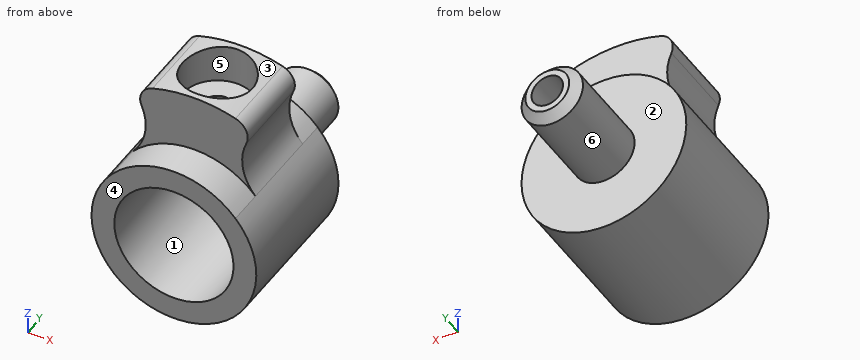
```python
from build123d import *

# Parameters (mm, degrees)
CUT_EXTRUDE_1_DEPTH   = 9.2
FILLET_1_R            = 1
SKETCH_5_OUTSIDE_W    = 15.602
SKETCH_5_OUTSIDE_H    = 18.902
SKETCH_5_OUTSIDE_R    = 4.7
CUT_EXTRUDE_4_DEPTH   = 1.5
CUT_EXTRUDE_START     = -8.2
SKETCH_5_2_OUTSIDE_W  = 15.602
SKETCH_5_2_OUTSIDE_H  = 18.902
SKETCH_5_2_OUTSIDE_R  = 4.7
CUT_EXTRUDE_5_DEPTH   = 2
CHAMFER_1_SIZE        = 0.5
M2_TAPPED_HOLE1_D     = 1.6
M2_TAPPED_HOLE1_DEPTH = 5.2
M2_TAPPED_HOLE1_TIP   = 0.480688495
SKETCH4_R             = 2
CUT_EXTRUDE1_DEPTH    = 2.2


with BuildPart() as part:
    # Эскиз1 → Повернуть1 (revolve)
    with BuildSketch(Plane(origin=(0, 0, 0), x_dir=(0, 0, -1), z_dir=(1, 0, 0))):
        Polygon((-3.4, 0), (-3.4, 6.5), (-0.9, 6.5), (-0.9, 13.85), (-1.75, 13.85), (-1.75, 8.2), (-8, 8.2), (-8, 0), align=None)
    revolve(axis=Axis((0, 0, 0), (0, 1, 0)))

    # Эскиз2 → Вырез-Вытянуть1 (cut, through all)
    with BuildSketch(Plane(origin=(0, 8.2, 0), x_dir=(1, 0, 0), z_dir=(0, 1, 0))):
        with BuildLine():
            ThreePointArc((7.99025974, -7.116582697), (0, 10.7), (-7.99025974, -7.116582697))
            ThreePointArc((-7.99025974, -7.116582697), (-3.75469644, -7.361538877), (-3.50974026, -3.125975577))
            ThreePointArc((-3.50974026, -3.125975577), (0, 4.7), (3.50974026, -3.125975577))
            ThreePointArc((3.50974026, -3.125975577), (3.75469644, -7.361538877), (7.99025974, -7.116582697))
        make_face()
    extrude(amount=-CUT_EXTRUDE_1_DEPTH, mode=Mode.SUBTRACT)

    # Скругление1
    fillet_1_edges = [part.edges().sort_by_distance(p)[0] for p in [
        (-3.555293146, 4.1, 7.166581517),
        (3.555293146, 4.1, 7.166581517),
    ]]
    fillet(fillet_1_edges, radius=FILLET_1_R)

    # Эскиз5 outside → Вырез-Вытянуть4 (cut)
    with BuildSketch(Plane(origin=(0, 8.2, 0), x_dir=(1, 0, 0), z_dir=(0, 1, 0))):
        with Locations((0, -1.65)):
            Rectangle(SKETCH_5_OUTSIDE_W, SKETCH_5_OUTSIDE_H)
        Circle(SKETCH_5_OUTSIDE_R, mode=Mode.SUBTRACT)
    extrude(amount=-CUT_EXTRUDE_4_DEPTH, mode=Mode.SUBTRACT)

    # Эскиз5<2> outside → Вырез-Вытянуть5 (cut)
    with BuildSketch(Plane(origin=(0, 8.2, 0), x_dir=(1, 0, 0), z_dir=(0, 1, 0)).offset(CUT_EXTRUDE_START)):
        with Locations((0, -1.65)):
            Rectangle(SKETCH_5_2_OUTSIDE_W, SKETCH_5_2_OUTSIDE_H)
        Circle(SKETCH_5_2_OUTSIDE_R, mode=Mode.SUBTRACT)
    extrude(amount=CUT_EXTRUDE_5_DEPTH, mode=Mode.SUBTRACT)

    # Фаска1
    chamfer_1_edges = [part.edges().sort_by_distance(p)[0] for p in [
        (0, 13.85, -1.75),
    ]]
    chamfer(chamfer_1_edges, length=CHAMFER_1_SIZE)

    # M2 Tapped Hole1
    with Locations(Plane(origin=(0, 8.2, 8), x_dir=(1, 0, 0), z_dir=(0, 0, 1))):
        with Locations((0, -3.85)):
            Hole(M2_TAPPED_HOLE1_D / 2, depth=M2_TAPPED_HOLE1_DEPTH)
            with Locations((0, 0, -(M2_TAPPED_HOLE1_DEPTH + M2_TAPPED_HOLE1_TIP / 2))):  # 118° drill point
                Cone(0, M2_TAPPED_HOLE1_D / 2, M2_TAPPED_HOLE1_TIP, mode=Mode.SUBTRACT)

    # Sketch4 → Cut-Extrude1 (cut)
    with BuildSketch(Plane(origin=(0, 8.2, 8), x_dir=(1, 0, 0), z_dir=(0, 0, 1))):
        with Locations((0, -3.85)):
            Circle(SKETCH4_R)
    extrude(amount=-CUT_EXTRUDE1_DEPTH, mode=Mode.SUBTRACT)


solid = part.part
```
Could you check a few things on this model? Use its own coordinates, in mm. Face numbers are marked on the shaded views. A direction names the side the tool comes from. Coordinates: 2 decimals unless noted, no trailing zeros. Loops run counter-clockwise (first coordinate to the right, second up) from the corner with the lowest first, then second, coordinate; pieces in that order, holes last.
1) Imagine slicing it at D-D (z = 2.5). List the corners of the cut face in (x, y) for me.
Reported:
outline: (-3.98, 0) - (-2.3, 0) - (-2.3, 6.5) - (2.3, 6.5) - (2.3, 0) - (3.98, 0) - (3.98, 8.2) - (-3.98, 8.2) - close
2) Please list where these lines run through material, in increasing order: line 1 along X through (y, z) = (3, 0); line 2 along X through (y, z) = (4.35, 6.6); line 3 along Y through (x, z) = (0, 7.3).
Reported:
line 1: x = -4.7 to -3.4, 3.4 to 4.7
line 2: x = -3.07 to -2, 2 to 3.07
line 3: y = 2 to 2.35, 6.35 to 6.7
3) Imagine slicing it at A-A (x = 0). State how many separate pieces and enclosed holes the cut face has, and give its area (3 significant figures).
Reported:
separate pieces: 3
enclosed holes: 0
area: 42.0 mm2
4) Will these pins go through, and if not, where does the flat tip stop? pin 1 Ø1.5 at (y, z) = (11, 3) entering from +X; pin 2 Ø4 at (x, z) = (0, 5) entering from +Y; pin 3 Ø1 at (x, y) = (0, 4.35) entering from +Z; pin 4 Ø3 at (x, y) = (-0.5, 11.5) entering from +Z.
Reported:
pin 1: passes through
pin 2: stops at y = 8.2
pin 3: stops at z = -3.36
pin 4: stops at z = 1.75
5) Imagine slicing it at B-B (z = 0). List the corners of the cut face in (x, y) for me, and give its area (3 significant figures).
Reported:
outline: (-4.7, 0) - (-3.4, 0) - (-3.4, 6.5) - (-0.9, 6.5) - (-0.9, 13.85) - (-1.25, 13.85) - (-1.75, 13.35) - (-1.75, 8.2) - (-4.7, 8.2) - close; (0.9, 6.5) - (3.4, 6.5) - (3.4, 0) - (4.7, 0) - (4.7, 8.2) - (1.75, 8.2) - (1.75, 13.35) - (1.25, 13.85) - (0.9, 13.85) - close
area: 39.2 mm2
6) Thinking about a two-plate mould opening in X: for the marked faces 4, 5 and 6, which applies, released by +X, released by -X, zero draft, split by the parting line, or undercut?
Reported:
face 4: zero draft
face 5: undercut
face 6: split by the parting line
7) Which directions (+Z, -Z, +X, -X, +Y, -Y) give clear straight access to the entire face, cutting with the end or side of a thin tool? Please do the marked faces 1, 2 and 3.
Reported:
face 1: -Y
face 2: +Y
face 3: +Z, +Y, -Y
8) Imagine slicing it at C-C (y = 11.5). List the corners of the cut face in (x, z) for me, and give its area (3 significant figures).
Reported:
outline: circle Ø3.5 at (0, 0); hole circle Ø1.8 at (0, 0)
area: 7.08 mm2
